Design review of the part built by this model. Coordinates are the model's own, in mm. Give positions to 0.01 mm unless a question says otherwise; leave off trailing zeros.
```python
from build123d import *

# Parameters (mm, degrees)
SKETCH1_R             = 65
BOSS_EXTRUDE1_DEPTH   = 10
FILLET1_R             = 1
F_6_32_TAPPED_HOLE1_D = 2.7051
F_8_CLEARANCE_HOLE1_D = 4.4958


with BuildPart() as part:
    # Sketch1 → Boss-Extrude1 (new body)
    with BuildSketch(Plane(origin=(0, 0, 0), x_dir=(1, 0, 0), z_dir=(0, 1, 0))):
        with Locations(Location((0, 0, 0), (0, 0, 270))):
            Circle(SKETCH1_R)
    extrude(amount=BOSS_EXTRUDE1_DEPTH)

    # Fillet1
    fillet1_edges = [part.edges().sort_by_distance(p)[0] for p in [
        (0, 0, -65),
        (0, 10, -65),
    ]]
    fillet(fillet1_edges, radius=FILLET1_R)

    # #6-32 Tapped Hole1 (through all)
    with Locations(Plane.XZ):
        with Locations((-46.445, 0), (46.445, 0), (-36.445, -13), (-36.445, 13), (36.445, 13), (36.445, -13), (10.00119449, -40.8), (0.00119449, -29.978097245), (-9.99880551, -40.8)):
            Hole(F_6_32_TAPPED_HOLE1_D / 2)

    # #8 Clearance Hole1 (through all)
    with Locations(Plane(origin=(0, 0, 0), x_dir=(-1, 0, 0), z_dir=(0, -1, 0))):
        with Locations((7.5, -7.5), (-7.5, -7.5), (7.5, 7.5), (-7.5, 7.5)):
            Hole(F_8_CLEARANCE_HOLE1_D / 2)


solid = part.part
```
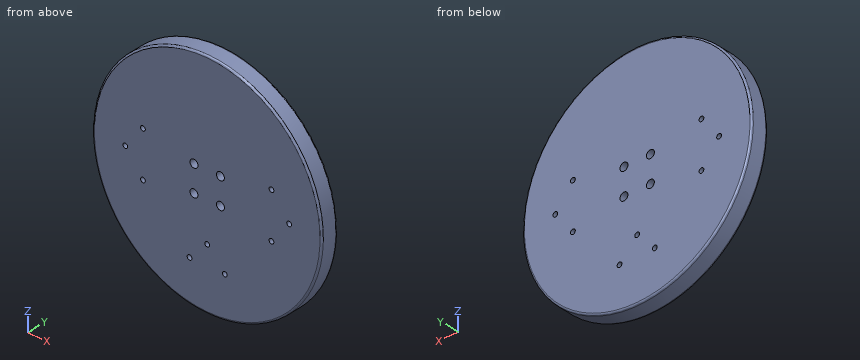
1. For pin 1 (1 mm diameter, centred on y = 4, z = 47.5, fed in from +X); pin 2 (3 mm diameter, centred on y = 6.5, z = -30.5, fed in from +X); pin 3 (1 mm diameter, centred on y = 7, z = 32.5, fed in from +X), all flat-tipped, find the tip position at first contact; note any pin that passes through.
Recorded:
pin 1: stops at x = 44.9
pin 2: stops at x = 58.17
pin 3: stops at x = 56.58
2. Take a section at A-A (y = 3.5). State how many separate pieces and enclosed holes the cut face has, then the cut area to 3 significant figures.
Recorded:
separate pieces: 1
enclosed holes: 13
area: 13,200 mm2
3. For line 1 along Z through (x, y) = (7.5, 2.5); line 2 along Z through (x, y) = (8.5, 1); line 3 along X through (y, z) = (6.75, -40.5), list the stretches that pass through material, from the lowest coordinate up.
Recorded:
line 1: z = -64.57 to -9.75, -5.25 to 5.25, 9.75 to 64.57
line 2: z = -64.44 to -9.51, -5.49 to 5.49, 9.51 to 64.44
line 3: x = -50.84 to -11.32, -8.68 to 8.68, 11.32 to 50.84
